Geometry: final body of the model. Coordinates: model frame, mm. A direction names the side the tool comes from. Give positions to 0.01 mm unless a question says otherwise; leave off trailing zeros. Write each loop counter-clockwise with the first axis right and the second up, starting at its lowest first coordinate (ties: lowest second). Pieces come first, ordered by that corner, then holes.
Q1. Cut plane D-D on y = 15. Count the separate pieces of the cut face and the enclosed holes in it, plus the area to 3 significant figures.
Q2. Draft query along Y for faces 3 (the face through (-31.21, -13.24, 0.18)), 4 (the face through (16, -11.913, 0)), 5 (the face through (28.1, 16, 0.2)), 6 (the face through (0, 0, -12.7)). Return one class per face: pulls with the +Y half, pulls with the -Y half, needs draft (parallel to the pull), parting line crosses it, or undercut.
Q3. Cut plane B-B on x = 3.5. Return the cut outline in (y, z).
Q4. Line query: L1, parallel to X at y = -4, z = 3.5 (3 decimals); L2, parallel to Y at x = 3, z = 5.25; L3, parallel to Y at x = 14.5, z = 5.75. Output: solid intervals per line, ascending.
Q5. Cut plane A-A on y = 3.5. Return the cut outline in (x, z) (3 decimals).
Q6. Pin query (flat end, axial travel): pin 1 (12.5 mm diameter, centred on x = -10.5, z = 3, fed in from +Y); pin 2 (8 mm diameter, centred on x = -8.5, y = -1, fed in from -Z). Return the tip coordinate at first contact, or that it passes through.
Q7. Reachability of faces 1 (the face through (-25.58, 13.145, 0.178)), 2 (the face through (31.18, -13.27, 0.18)) from +Z, -Z, +X, -X, +Y, -Y: full face, straight path, thin tool, end or side. Return the list, or none.
```python
from build123d import *

# Parameters (mm, degrees)
BASE_EXTRUDE_DEPTH = 12.7
LPATTERN1_COUNT    = 2
LPATTERN1_PITCH    = 31.75


with BuildPart() as part:
    # Sketch1 → Base-Extrude (new, symmetric)
    with BuildSketch(Plane.XY):
        with BuildLine():
            Line((-31.75, 14.335125), (-31.75, -11.9126))
            ThreePointArc((-31.75, -11.9126), (-31.192038418, -13.259638418), (-29.845, -13.8176))
            Line((-29.845, -13.8176), (-1.905, -13.8176))
            ThreePointArc((-1.905, -13.8176), (-0.557961582, -13.259638418), (0, -11.9126))
            Line((0, -11.9126), (0, 14.335125))
            ThreePointArc((0, 14.335125), (-3.571875, 17.907), (-7.14375, 14.335125))
            Line((-7.14375, 14.335125), (-7.14375, 14.097))
            ThreePointArc((-7.14375, 14.097), (-6.19125, 13.1445), (-5.23875, 14.097))
            Line((-5.23875, 14.097), (-5.23875, 14.335125))
            ThreePointArc((-5.23875, 14.335125), (-3.571875, 16.002), (-1.905, 14.335125))
            Line((-1.905, 14.335125), (-1.905, -11.9126))
            Line((-1.905, -11.9126), (-29.845, -11.9126))
            Line((-29.845, -11.9126), (-29.845, 14.335125))
            ThreePointArc((-29.845, 14.335125), (-28.178125, 16.002), (-26.51125, 14.335125))
            Line((-26.51125, 14.335125), (-26.51125, 14.097))
            ThreePointArc((-26.51125, 14.097), (-25.55875, 13.1445), (-24.60625, 14.097))
            Line((-24.60625, 14.097), (-24.60625, 14.335125))
            ThreePointArc((-24.60625, 14.335125), (-28.178125, 17.907), (-31.75, 14.335125))
        make_face()
    base_extrude = extrude(amount=BASE_EXTRUDE_DEPTH, both=True)

    # LPattern1: Base-Extrude ×2
    with Locations(*[(i * LPATTERN1_PITCH, 0, 0) for i in range(1, LPATTERN1_COUNT)]):
        add(base_extrude)


solid = part.part
```
Data:
1. separate pieces: 8
1. enclosed holes: 0
1. area: 403 mm2
2. face 3: pulls with the -Y half
2. face 4: undercut
2. face 5: undercut
2. face 6: needs draft
3. outline: (-13.82, -12.7) - (-11.91, -12.7) - (-11.91, 12.7) - (-13.82, 12.7) - close; (16, -12.7) - (17.91, -12.7) - (17.91, 12.7) - (16, 12.7) - close
4. L1: x = -31.75 to -29.845, -1.905 to 1.905, 29.845 to 31.75
4. L2: y = -13.82 to -11.91, 15.9 to 17.86
4. L3: y = -13.82 to -11.91
5. outline: (-31.75, -12.7) - (-29.845, -12.7) - (-29.845, 12.7) - (-31.75, 12.7) - close; (-1.905, -12.7) - (1.905, -12.7) - (1.905, 12.7) - (-1.905, 12.7) - close; (29.845, -12.7) - (31.75, -12.7) - (31.75, 12.7) - (29.845, 12.7) - close
6. pin 1: stops at y = 17.84
6. pin 2: passes through
7. face 1: +Z, -Z
7. face 2: +Z, -Z, +X, -Y
